Autodesk Inventor part; units mm, degrees
ref_plane "Work Plane3" through (-25, 0, 42.5) normal (0, -1, 0) x (1, 0, 0)
ref_plane "YZ Plane" through (0, 0, 0) normal (1, 0, 0) x (0, 1, 0)
ref_plane "XZ Plane" through (0, 0, 0) normal (0, 1, 0) x (-1, 0, 0)
ref_plane "Work Plane3" through (-25, 0, 42.5) normal (0, -1, 0) x (1, 0, 0)
sketch "Sketch1" plane through (-25, 0, 42.5) normal (0, -1, 0) x (1, 0, 0)
  line L0 (28.4781, -19.558) -> (28.4781, -33.5534)
  arc A0 (53, -3) -> (50, 0) centre (50, -3) ccw
  line L1 (0, 0) -> (50, 0)
  arc A1 (0, 0) -> (-3, -3) centre (0, -3) ccw
  line L2 (-3, -82) -> (-3, -3)
  arc A2 (-3, -82) -> (0, -85) centre (0, -82) ccw
  line L3 (50, -85) -> (0, -85)
  arc A3 (50, -85) -> (53, -82) centre (50, -82) ccw
  line L4 (53, -3) -> (53, -82)
  circle A4 centre (49.5, -61.5) radius 1.75
  circle A5 centre (0.5, -61.5) radius 1.75
  circle A6 centre (0.5, -3.5) radius 1.75
  circle A7 centre (49.5, -3.5) radius 1.75
  line L5 (-3, 0) -> (53, 0)
  line L6 (53, 0) -> (53, -88.9)
  line L7 (53, -88.9) -> (-3, -88.9)
  line L8 (-3, -88.9) -> (-3, 0)
  point P0 (25, -42.5)
  dimension "d0" = 88.9
extrude "Extrusion1" add sketch "Sketch1" along normal blind 3.175
sketch "Sketch2" plane through (-25, -3.175, 42.5) normal (0, -1, 0) x (1, 0, 0)
  circle A0 centre (49.5, -3.5) radius 1.75
  circle A1 centre (0.5, -3.5) radius 1.75
  circle A2 centre (0.5, -61.5) radius 1.75
  circle A3 centre (49.5, -61.5) radius 1.75
  line L0 (53, 0) -> (-3, 0)
  line L1 (-3, 0) -> (-3, -88.9)
  line L2 (-3, -88.9) -> (53, -88.9)
  line L3 (53, -88.9) -> (53, 0)
  line L4 (-3, -88.9) -> (53, -88.9)
  line L5 (55.8, 2.8) -> (55.8, -91.7)
  line L6 (-5.8, -91.7) -> (-5.8, 2.8)
  line L7 (53, 0) -> (55.8, 2.8)
  line L8 (53, 0) -> (58.3967, 0) construction
  line L9 (55.8, 2.8) -> (-5.8, 2.8)
  line L10 (53, -88.9) -> (61.5609, -88.9) construction
  line L11 (55.8, -91.7) -> (-5.8, -91.7)
  point P0 (25, -42.5)
  dimension "d3" = 45
extrude "Extrusion2" add sketch "Sketch2" against normal blind 3.175 contours L5 L11 L6 L9
sketch "Sketch3" plane through (-25, 0, 42.5) normal (0, 1, 0) x (1, 0, 0)
  line L0 (-5.8, -2.8) -> (55.8, -2.8)
  line L1 (55.8, -2.8) -> (55.8, 91.7)
  line L2 (55.8, 91.7) -> (-5.8, 91.7)
  line L3 (-5.8, 91.7) -> (-5.8, -2.8)
  line L4 (53, 3.55) -> (55.8, 3.55)
  line L5 (55.8, 3.55) -> (55.8, 85.35)
  line L6 (55.8, 85.35) -> (53, 85.35)
  line L7 (53, 85.35) -> (53, 3.55)
  point P0 (25, 42.5)
  dimension "d7" = 6.35
  dimension "d20" = 6.35
extrude "Extrusion3" cut sketch "Sketch3" against normal blind 15.875 contours L4 L7 L6 L1
sketch "Sketch5" plane through (-25, 0, 42.5) normal (0, 1, 0) x (1, 0, 0)
  line L0 (-3, 88.9) -> (16.05, 88.9)
  line L1 (16.05, 88.9) -> (16.05, 91.7575)
  line L2 (16.05, 91.7575) -> (-3, 91.7575)
  line L3 (-3, 91.7575) -> (-3, 88.9)
  line L4 (55.8, 3.55) -> (53, 3.55)
  line L5 (53, 85.35) -> (55.8, 85.35)
  line L6 (55.8, 85.35) -> (55.8, 91.7)
  line L7 (55.8, 91.7) -> (-5.8, 91.7)
  line L8 (-5.8, 91.7) -> (-5.8, -2.8)
  line L9 (-5.8, -2.8) -> (55.8, -2.8)
  line L10 (55.8, -2.8) -> (55.8, 3.55)
  line L11 (53, 3.55) -> (53, 85.35)
  point P0 (25, 42.5)
  dimension "d15" = 19.05
  dimension "d16" = 2.8575
extrude "Extrusion5" cut sketch "Sketch5" against normal blind 15.875 contours L3 L7 L1 L0 | L3 L2 L1 L7
sketch "Sketch6" plane through (-25, -3.175, 42.5) normal (0, -1, 0) x (1, 0, 0)
  line L0 (16.05, -88.9) -> (16.05, -91.7)
  line L1 (16.05, -91.7) -> (55.8, -91.7)
  line L2 (55.8, -91.7) -> (55.8, -85.35)
  line L3 (55.8, -85.35) -> (53, -85.35)
  line L4 (53, -85.35) -> (53, -3.55)
  line L5 (53, -3.55) -> (55.8, -3.55)
  line L6 (55.8, -3.55) -> (55.8, 2.8)
  line L7 (55.8, 2.8) -> (-5.8, 2.8)
  line L8 (-5.8, 2.8) -> (-5.8, -91.7)
  line L9 (-5.8, -91.7) -> (-3, -91.7)
  line L10 (-3, -91.7) -> (-3, -88.9)
  line L11 (-3, -88.9) -> (16.05, -88.9)
  circle A0 centre (49.5, -61.5) radius 1.75
  circle A1 centre (0.5, -61.5) radius 1.75
  circle A2 centre (0.5, -3.5) radius 1.75
  circle A3 centre (49.5, -3.5) radius 1.75
  line L12 (34.525, 2.8) -> (34.525, -0.0575)
  line L13 (16.05, -88.9) -> (-3, -88.9)
  line L14 (16.05, -0.0575) -> (15.475, -0.0575)
  line L15 (15.475, -0.0575) -> (15.475, -88.9)
  line L16 (15.475, -88.9) -> (16.05, -88.9)
  line L17 (34.525, -88.9) -> (34.525, -0.0575)
  line L18 (16.05, -91.7) -> (55.8, -91.7)
  line L19 (16.05, -88.9) -> (16.05, -91.7)
  line L20 (16.05, -91.7) -> (34.525, -91.7)
  line L21 (34.525, -91.7) -> (34.525, -88.9)
  line L22 (15.475, -0.0575) -> (16.05, -0.0575)
  line L23 (34.525, -0.0575) -> (34.525, 2.8)
  line L24 (34.525, 2.8) -> (15.475, 2.8)
  line L25 (15.475, 2.8) -> (15.475, -0.0575)
  point P0 (25, -42.5)
extrude "Extrusion6" add sketch "Sketch6" along normal blind 9.525 contours L11 L15 L25 L7 L12 L17 L21 L1 L0
chamfer "Chamfer1" distance 3.175 angle 45 2 edges at (-9.525, -3.175, -0.55) (9.525, -3.175, -1.95)
chamfer "Chamfer2" distance 3.175 angle 45 2 edges at (9.525, -6.35, -1.95) (-9.525, -6.35, -0.55)
chamfer "Chamfer3" distance 3.175 angle 45 2 edges at (9.525, -12.7, -1.95) (-9.525, -12.7, -0.55)
fillet "Fillet1" radius 3.175 2 edges at (-12.7, -3.175, -0.55) (12.7, -3.175, -1.95)
properties part number "Raspi3B+_Case"
For this review, take the finished solid that the model builds, in its own axes (mm). A direction names the side the tool comes from. Give positions to 0.01 mm unless a question says otherwise; leave off trailing zeros. Loops run counter-clockwise (first coordinate to the right, second up) from the corner with the lowest first, then second, coordinate; pieces in that order, holes last. Notation, with made-up numbers: M -8.5,66 L 41.5,66 A28 cw 41.5,101 Z; hole C 71,85 d11. An arc over 180 degrees is marked long. Put each result on its own line as item: value. Start each with the question number.
(1) Machinability: for faces 1 (the flat face through (22, -3.175, -1)), 2 (the flat face through (0, -12.7, -1)), 3 (the flat face through (28, -2, -3)), 4 (the cylindrical face through (-25.89, -1.57, 40.06)), 5 (the flat face through (-23, -3.175, -1)), which of the approach directions +Z, -Z, +X, -X, +Y, -Y give a long, thin tool a straight path to every point of the face, cutting with its end or side? Answer none if there is none.
(2) Add section D-D, the plane y = -11.25. Write out the cut boundary in (x, z), then the cut area to 3 significant figures.
(3) Wall thickness on L1, parallel to Z at x = -24.5, y = -1.85; L2, parallel to Y at x = -27.5, z = 15 (3 decimals); L3, parallel to X at y = -0.25, z = 14: over which ranges is each line inside the solid? List them lowest first.
(4) Add section C-C, the plane x = 24.5. Write out the cut boundary in (y, z) (3 decimals), then the cut area to 3 significant figures.
(5) For pin 1 (5.5 mm diameter, centred on x = -24.5, z = 39, fed in from -Y) (3 decimals); pin 2 (3 mm diameter, centred on x = -24.5, z = -19, fed in from -Y); pin 3 (18.5 mm diameter, centred on x = 22.5, z = -3, fed in from -Y); pin 4 (2 mm diameter, centred on y = -5.5, z = 12.5, fed in from -X), all flat-tipped, find the tip position at first contact; note any pin that passes through.
(6) Add section A-A, the plane x = -24.5. Write out the cut boundary in (y, z) (3 decimals).
(7) The part is to be moulded in two halves that separate along X. For faces 6 (the cylindrical face through (-12.82, -3.41, -1.19)), 7 (the flat face through (0, -5, 45.3)), 8 (the flat face through (-28, -2, -48)), say which applies: +X half, -X half, draft (parallel to the pull), parting line (faces both ways), or undercut.
Result:
1. face 1: +Z, -Z, +X, -Y
1. face 2: +Z, -Z, +X, -X, -Y
1. face 3: +X, +Y, -Y
1. face 4: +Y, -Y
1. face 5: +Z, -Z, -X, -Y
2. outline: M -7.8,-49.2 L 7.8,-49.2 L 7.8,45.3 L -7.8,45.3 Z
2. area: 1,470 mm^2
3. L1: z = -46.4 to -20.75, -17.25 to 37.25, 40.75 to 45.3
3. L2: y = -3.175 to 0
3. L3: x = -30.8 to 28
4. outline: M -3.175,-49.2 L 0,-49.2 L 0,-20.75 L -3.175,-20.75 Z; M -3.175,-17.25 L 0,-17.25 L 0,37.25 L -3.175,37.25 Z; M -3.175,40.75 L 0,40.75 L 0,45.3 L -3.175,45.3 Z
4. area: 278 mm^2
5. pin 1: stops at y = -3.175
5. pin 2: passes through
5. pin 3: stops at y = -3.27
5. pin 4: stops at x = -11.61
6. outline: M -3.175,-46.4 L 0,-46.4 L 0,-20.75 L -3.175,-20.75 Z; M -3.175,-17.25 L 0,-17.25 L 0,37.25 L -3.175,37.25 Z; M -3.175,40.75 L 0,40.75 L 0,45.3 L -3.175,45.3 Z
7. face 6: -X half
7. face 7: draft
7. face 8: undercut
